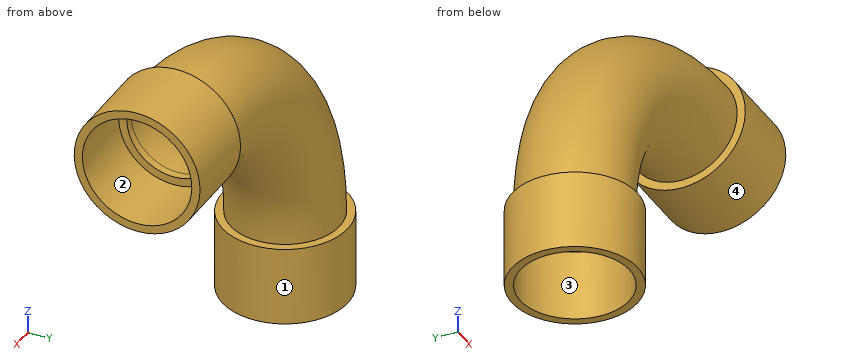
Autodesk Inventor part; units mm, degrees
ref_plane "YZ Plane" through (0, 0, 0) normal (1, 0, 0) x (0, 1, 0)
ref_plane "XZ Plane" through (0, 0, 0) normal (0, 1, 0) x (-1, 0, 0)
ref_plane "XY Plane" through (0, 0, 0) normal (0, 0, 1) x (1, 0, 0)
sketch "Sketch1" plane through (0, 0, 0) normal (0, 1, 0) x (-1, 0, 0)
  line L0 (0, 0) -> (0, 29)
  line L1 (17, 29) -> (23, 29)
  line L2 (0, 29) -> (17, 29) construction
  line L3 (23, 29) -> (23, 0)
  line L4 (23, 0) -> (20, 0)
  line L5 (20, 0) -> (20, 26)
  line L6 (20, 0) -> (0, 0) construction
  line L7 (-106, 106) -> (-77, 106)
  line L8 (-77, 106) -> (-77, 89) construction
  line L9 (-106, 83) -> (-106, 86)
  line L10 (-106, 86) -> (-80, 86)
  line L11 (-106, 86) -> (-106, 106) construction
  line L12 (-77, 106) -> (0, 106) construction
  line L13 (0, 106) -> (0, 29) construction
  line L14 (17, 29) -> (17, 26)
  line L15 (17, 26) -> (20, 26)
  line L16 (-77, 89) -> (-80, 89)
  line L17 (-80, 89) -> (-80, 86)
  line L18 (-106, 83) -> (-77, 83)
  line L19 (-77, 89) -> (-77, 83)
  line L20 (-80, 89) -> (-80, 106) construction
  line L21 (17, 26) -> (0, 26) construction
  dimension "d0" = 40
  dimension "d1" = 3
  dimension "d2" = 26
  dimension "d4" = 34
  dimension "d6" = 40
  dimension "d7" = 34
  dimension "d10" = 3
  dimension "d11" = 3
  dimension "d12" = 26
  dimension "d14" = 80
  dimension "d15" = 80
  dimension "d16" = 3
revolve "Revolution1" add sketch "Sketch1" angle 360 about axis through (0, 0, 0) along (0, 0, 1) contours L1 L3 L4 L5 L15 L14
sketch "Sketch2" plane through (0, 0, 0) normal (0, 1, 0) x (-1, 0, 0)
  line L0 (0, 29) -> (0, 106) construction
  line L1 (0, 106) -> (-77, 106) construction
  arc A0 (0, 29) -> (-77, 106) centre (-77, 29) ccw
  line L2 (-23, 29) -> (23, 29)
  dimension "d8" = 77
  dimension "d9" = 77
sketch "Sketch3" plane through (0, 0, 29) normal (0, 0, 1) x (1, 0, 0)
  circle A0 centre (0, 0) radius 20
  circle A1 centre (0, 0) radius 20
  circle A2 centre (0, 0) radius 17
  circle A3 centre (0, 0) radius 17
  dimension "d13" = 40
sweep "Sweep1" add profiles "Sketch3" path "Sketch2" path curves A0
revolve "Revolution2" add sketch "Sketch1" angle 360 about axis through (106, 0, 106) along (-1, 0, 0) contours L9 L10 L17 L16 L19 L18
equation "\"d0\" = D1"
equation "\"d1\" = S"
equation "\"d2\" = T"
equation "\"d4\" = D1 - 2 * S"
equation "\"d6\" = D1"
equation "\"d7\" = D1 - 2 * S"
equation "\"d10\" = S"
equation "\"d11\" = S"
equation "\"d12\" = T"
equation "\"d14\" = Z"
equation "\"d15\" = Z"
equation "\"d16\" = S"
equation "\"d8\" = Z - S"
equation "\"d9\" = Z - S"
equation "\"d13\" = D1"
equation "\"D1\" = 40"
equation "\"T\" = 26"
equation "\"Z\" = 80"
equation "\"S\" = 3"
properties part number "DIN 8063 Колено 90 градусов, тип B 40" material "ПВХ, непластифицированный"
Here's how the part is built. I have some questions about the finished solid (model axes, mm). Face numbers are marked on the shaded views. A direction names the side the tool comes from. Give positions to 0.01 mm unless a question says otherwise; leave off trailing zeros. Order: outer loops, then holes, each group sorted by start corner. A loop starts at its lowest first (then second) coordinate and runs counter-clockwise, first axis right, second up. Notation, with made-up numbers: M -9.5,86 L 42.5,86 A25 ccw 42.5,102 Z; hole C 80.25,69.25 d6. An arc over 180 degrees is marked long. Use a Markdown table: item, result. Add a question column.
1. Suppose I cut it at B-B (z = 10.5). List the corners of the cut face in (x, y) for me.
2. On a 3-axis mill with a long thin cutter (end or side, diameter ignored), from which of +Z, -Z, +X, -X, +Y, -Y can I reach the whole of each face in a straight line? I mean the marked faces 3 and 4. Say none if no direction works.
3. Suppose I cut it at C-C (x = 95). List the corners of the cut face in (y, z) for me.
4. Suppose I cut it at A-A (y = 0). List the corners of the cut face in (x, z) for me, and give its area (3 significant figures).
5. Suppose I cut it at D-D (y = 7). List the corners of the cut face in (x, z) for me (3 decimals).
6. For pin 1 Ø20 at (x, y) = (5.5, 1.5) entering from -Z; pin 2 Ø5 at (x, y) = (-5.5, 10) entering from +Z; pin 3 Ø6 at (y, z) = (16, 108.5) entering from -X, each with a flat end and sliding along its axis, tell me the tip position at first contact or that it passes through.
7. If we mould it in two halves opening along Y, with no side actions, what happens to the marked faces 1 and 2? For each: +Y half, -Y half, draft (parallel to the pull), parting line (faces both ways), or undercut.
8. I need wall thicknesses on probe 1 along X at (y, z) = (0, 10.25); probe 2 along Y at (x, z) = (79.2, 106). Which ranges of each line are inside material? Lowest first, please. Write a range as from..to.
Results list:
| question | item | result |
|---|---|---|
| 1 | outline | C 0,0 d46; hole C 0,0 d40 |
| 2 | face 3 | -Z |
| 2 | face 4 | +X |
| 3 | outline | C 0,106 d46; hole C 0,106 d40 |
| 4 | outline | M -23,0 L -20,0 L -20,26 L -17,26 L -17,29 A94 cw 77,123 L 80,123 L 80,126 L 106,126 L 106,129 L 77,129 L 77,126 A97 ccw -20,29 L -23,29 Z; M 17,26 L 20,26 L 20,0 L 23,0 L 23,29 L 20,29 A57 cw 77,86 L 77,83 L 106,83 L 106,86 L 80,86 L 80,89 L 77,89 A60 ccw 17,29 Z |
| 4 | area | 1,110 mm² |
| 5 | outline | M -21.909,0 L -18.735,0 L -18.735,26 L -15.492,26 L -15.492,29 A92.492 cw 77,121.492 L 80,121.492 L 80,124.735 L 106,124.735 L 106,127.909 L 77,127.909 L 77,124.735 A95.735 ccw -18.735,29 L -21.909,29 Z; M 15.492,26 L 18.735,26 L 18.735,0 L 21.909,0 L 21.909,29 L 18.735,29 A58.265 cw 77,87.265 L 77,84.091 L 106,84.091 L 106,87.265 L 80,87.265 L 80,90.508 L 77,90.508 A61.508 ccw 15.492,29 Z |
| 6 | pin 1 | stops at z = 75.42 |
| 6 | pin 2 | stops at z = 79.68 |
| 6 | pin 3 | stops at x = 28.34 |
| 7 | face 1 | parting line |
| 7 | face 2 | undercut |
| 8 | probe 1 | x = -23..-20, 20..23 |
| 8 | probe 2 | y = -23..-17, 17..23 |
